```python
from build123d import *

# Parameters (mm, degrees)
SZKIC1_R                    = 12
DODANIE_WYCI_GNI_CIE1_DEPTH = 5
WYTNIJ_WYCI_GNI_CIE1_START  = -5
WYTNIJ_WYCI_GNI_CIE1_DEPTH  = 5
SZYK_KO_OWY1_COUNT          = 3
ZAOKR_GLENIE1_R             = 0.5
SZKIC4_R                    = 5.5
DODANIE_WYCI_GNI_CIE2_DEPTH = 3
SZKIC5_R                    = 2.5
DODANIE_WYCI_GNI_CIE3_DEPTH = 18
ZAOKR_GLENIE2_R             = 1
SFAZOWANIE1_SIZE            = 0.3


with BuildPart() as part:
    # Szkic1 → Dodanie-wyciągnięcie1 (new body)
    with BuildSketch(Plane(origin=(0, 0, 0), x_dir=(1, 0, 0), z_dir=(0, 1, 0))):
        with Locations(Location((0, 0, 0), (0, 0, 270))):
            Circle(SZKIC1_R)
    extrude(amount=DODANIE_WYCI_GNI_CIE1_DEPTH)

    # Szkic2 → Wytnij-wyciągnięcie1 (cut)
    with BuildSketch(Plane(origin=(0, 5, 0), x_dir=(1, 0, 0), z_dir=(0, 1, 0)).offset(WYTNIJ_WYCI_GNI_CIE1_START)):
        with BuildLine():
            ThreePointArc((-11.736670864, -2.500111405), (-5.986418703, -10.400134187), (3.732985364, -11.404596454))
            ThreePointArc((3.732985364, -11.404596454), (-2.820371946, -4.899798719), (-11.736670864, -2.500111405))
        make_face()
    wytnij_wyci_gni_cie1 = extrude(amount=WYTNIJ_WYCI_GNI_CIE1_DEPTH, mode=Mode.SUBTRACT)

    # Szyk kołowy1: Wytnij-wyciągnięcie1 ×3 about axis
    szyk_ko_owy1_axis = Axis((0, 0, 0), (0, 1, 0))
    for i in range(1, SZYK_KO_OWY1_COUNT):
        add(wytnij_wyci_gni_cie1.rotate(szyk_ko_owy1_axis, i * 360 / SZYK_KO_OWY1_COUNT), mode=Mode.SUBTRACT)

    # Szkic3 → Wycięcie-obrót2 (revolve, cut)
    with BuildSketch(Plane.XY, mode=Mode.PRIVATE) as wyci_cie_obr_t2_sk:
        with BuildLine():
            Line((0, 0), (0, -1))
            Line((0, -1), (-12, -1))
            Line((-12, -1), (-12, 3.560911085))
            ThreePointArc((-12, 3.560911085), (-6.258595844, 0.909007182), (0, 0))
        make_face()
    revolve(wyci_cie_obr_t2_sk.sketch.rotate(Axis((0, -5.338346039, 0), (0, 1, 0)), 180), axis=Axis((0, -5.338346039, 0), (0, 1, 0)), mode=Mode.SUBTRACT)

    # Zaokrąglenie1
    zaokr_glenie1_edges = [part.edges().sort_by_distance(p)[0] for p in [
        (3.703175443, 4.280455543, -11.414310826),
        (-11.743162931, 4.280455543, -2.469438069),
        (-2.833164191, 0.738827064, -4.892413113),
        (8.033495421, 4.280455543, 8.914199421),
        (8.010177567, 4.280455543, -8.935158384),
        (-11.736670864, 4.280455543, 2.500111405),
        (3.732985364, 4.280455543, 11.404596454),
        (6.013571057, 3.560911085, 10.384457768),
        (5.986418703, 3.560911085, -10.400134187),
        (-2.820371946, 0.738827064, 4.899798719),
        (6.315413129, 1.481143646, 4.805423076),
        (-11.99998976, 3.560911085, 0.015676419),
    ]]
    fillet(zaokr_glenie1_edges, radius=ZAOKR_GLENIE1_R)

    # Szkic4 → Dodanie-wyciągnięcie2 (add)
    with BuildSketch(Plane(origin=(0, 5, 0), x_dir=(1, 0, 0), z_dir=(0, 1, 0))):
        with Locations(Location((0, 0, 0), (0, 0, 270))):
            Circle(SZKIC4_R)
    extrude(amount=DODANIE_WYCI_GNI_CIE2_DEPTH)

    # Szkic5 → Dodanie-wyciągnięcie3 (add)
    with BuildSketch(Plane(origin=(0, 8, 0), x_dir=(1, 0, 0), z_dir=(0, 1, 0))):
        with Locations(Location((0, 0, 0), (0, 0, 270))):
            Circle(SZKIC5_R)
    extrude(amount=DODANIE_WYCI_GNI_CIE3_DEPTH)

    # Zaokrąglenie2
    # the kernel refuses this fillet: 1 mm, written as the material it adds along each edge
    with BuildSketch(Plane(origin=(0, 5, 0), x_dir=(0, 0, 1), z_dir=(-1, 0, 0))) as zaokr_glenie2_piece_1_section:
        with BuildLine():
            CenterArc((5.5 + ZAOKR_GLENIE2_R, ZAOKR_GLENIE2_R), ZAOKR_GLENIE2_R, 180, 90)
            Line((5.5, ZAOKR_GLENIE2_R), (5.5, 0))
            Line((5.5, 0), (5.5 + ZAOKR_GLENIE2_R, 0))
        make_face()
    zaokr_glenie2_piece_1 = revolve(axis=Axis((0, 5, 0), (0, 1, 0)), mode=Mode.PRIVATE)
    zaokr_glenie2_piece_1 = zaokr_glenie2_piece_1 - Plane(origin=(-11.8, 5.278674407, 20.5), x_dir=(0.8629436313514112, 0, -0.5053001970215725), z_dir=(0, -1, 0)) * Cylinder(18, 26, mode=Mode.PRIVATE)
    zaokr_glenie2_piece_1 = zaokr_glenie2_piece_1 - Plane(origin=(23.653520778, 5.278674407, -0.030900235), x_dir=(-0.8690746228336692, 0, -0.49468100827352957), z_dir=(0, -1, 0)) * Cylinder(18, 26, mode=Mode.PRIVATE)
    zaokr_glenie2_piece_1 = zaokr_glenie2_piece_1 - Plane(origin=(-11.853520778, 5.278674407, -20.469099765), x_dir=(0.006130991482257597, 0, 0.9999812052951018), z_dir=(0, -1, 0)) * Cylinder(18, 26, mode=Mode.PRIVATE)
    add(zaokr_glenie2_piece_1)

    # Sfazowanie1
    sfazowanie1_edges = [part.edges().sort_by_distance(p)[0] for p in [
        (0, 26, -2.5),
    ]]
    chamfer(sfazowanie1_edges, length=SFAZOWANIE1_SIZE)


solid = part.part
```
Geometry: final body of the model. Coordinates: model frame, mm. A direction names the side the tool comes from. Coordinates: 2 decimals unless noted, no trailing zeros. Put each result on its own line as item: value.
(1) Material intervals for probe 1 along Y at (x, z) = (3, -6.25); probe 2 along X at (y, z) = (8.5, 2), sorted ascending.
Answer sheet:
probe 1: y = 1.12 to 5
probe 2: x = -1.5 to 1.5
(2) First-contact query: pin 1 (10 mm diameter, centred on x = -6, z = 4.5, fed in from -Y); pin 2 (1 mm diameter, centred on x = 3.5, y = 9.5, fed in from -Z); pin 3 (6.5 mm diameter, centred on x = 5.5, z = -6, fed in from +Y); pin 4 (6 mm diameter, centred on y = 6, z = -9, fed in from +X). Flat tips, straight axial feed; report the tip coordinate or a pass-through.
Answer sheet:
pin 1: stops at y = 0.14
pin 2: passes through
pin 3: stops at y = 8
pin 4: stops at x = 7.88
(3) Access query for faces 1 (the face through (5, 5, -8)), 2 (the face through (5, 5, 8)), 3 (the face through (0, 8, -3)). Directions: +Z, -Z, +X, -X, +Y, -Y. A direction counts if a zero-diameter tool reaches every point of the face in a straight line with its end or side. Return the directions, or none.
Answer sheet:
face 1: -Z, +X, +Y
face 2: +Z, +X, +Y
face 3: +Y
